Source: CAD feature listing. Evaluate the final solid. Frame: model axes, mm. Give positions to 0.01 mm unless a question says otherwise; leave off trailing zeros. Loops run counter-clockwise (first coordinate to the right, second up) from the corner with the lowest first, then second, coordinate; pieces in that order, holes last. Notation, with made-up numbers: M -2,48.25 L 18,48.25 A15 ccw 18,72.25 Z; hole C 10.25,22 d5. An arc over 180 degrees is marked long. Write item = value, one per line.
from build123d import *

# Parameters (mm, degrees)
SKETCH2_R           = 2
SKETCH2_R_2         = 4.0005
BOSS_EXTRUDE1_DEPTH = 6.35


with BuildPart() as part:
    # Sketch2 → Boss-Extrude1 (new body)
    with BuildSketch(Plane(origin=(0, 0, 0), x_dir=(1, 0, 0), z_dir=(0, 1, 0))):
        with BuildLine():
            Line((6.35, 127), (12.7, 127))
            ThreePointArc((12.7, 127), (21.680256121, 123.280256121), (25.4, 114.3))
            Line((25.4, 114.3), (25.4, 101.6))
            Line((25.4, 101.6), (15.875, 92.075))
            Line((15.875, 92.075), (6.35, 92.075))
            Line((6.35, 92.075), (6.35, 101.6))
            Line((6.35, 101.6), (6.35, 127))
        make_face()
        with Locations((11.43, 97.155)):
            Circle(SKETCH2_R, mode=Mode.SUBTRACT)
        with Locations((19.05, 104.14)):
            Circle(SKETCH2_R, mode=Mode.SUBTRACT)
        with Locations((12.7, 114.3)):
            Circle(SKETCH2_R_2, mode=Mode.SUBTRACT)
    extrude(amount=BOSS_EXTRUDE1_DEPTH)


solid = part.part
1. Cut plane B-B, the plane x = 19.05. Return the cut outline in (y, z).
Derived:
outline = M 0,-125.3 L 6.35,-125.3 L 6.35,-106.14 L 0,-106.14 Z; M 0,-102.14 L 6.35,-102.14 L 6.35,-95.25 L 0,-95.25 Z
2. Cut plane C-C, the plane y = 3. Count the separate pieces of the cut face and the enclosed holes in it, then the cut area to 3 significant figures.
Derived:
separate_pieces = 1
enclosed_holes = 3
area = 510 mm²
3. Cut plane A-A, the plane z = -104.14. Return the cut outline in (x, y), then the cut area to 3 significant figures.
Derived:
outline = M 6.35,0 L 17.05,0 L 17.05,6.35 L 6.35,6.35 Z; M 21.05,0 L 25.4,0 L 25.4,6.35 L 21.05,6.35 Z
area = 95.6 mm²
4. Cut plane D-D, the plane x = 11.43. Return the cut outline in (y, z) (3 decimals), then the cut area to 3 significant figures.
Derived:
outline = M 0,-127 L 6.35,-127 L 6.35,-118.094 L 0,-118.094 Z; M 0,-110.506 L 6.35,-110.506 L 6.35,-99.155 L 0,-99.155 Z; M 0,-95.155 L 6.35,-95.155 L 6.35,-92.075 L 0,-92.075 Z
area = 148 mm²
5. Pull-direction query (X, two-part tool) for faces 1 (the flat face through (16, 6.35, -110)), 2 (the cylindrical face through (18.616, 3.131, -102.188)), 3 (the flat face through (20.7, 3.1, -96.9)); classes: +X half, -X half, draft (parallel to the pull), parting line (faces both ways), or undercut.
Derived:
face_1 = draft
face_2 = undercut
face_3 = +X half
6. Material intervals for probe 1 along X at (y, z) = (4.75, -104.14); probe 2 along Z at (x, y) = (12.7, 5) (1 decimal); probe 3 along Z at (x, y) = (11.43, 3.75) (3 decimals), sorted ascending. Write a range as from..to.
Derived:
probe_1 = 6.35..17.05, 21.05..25.4
probe_2 = -127..-118.3, -110.3..-98.7, -95.6..-92.1
probe_3 = -127..-118.094, -110.506..-99.155, -95.155..-92.075
